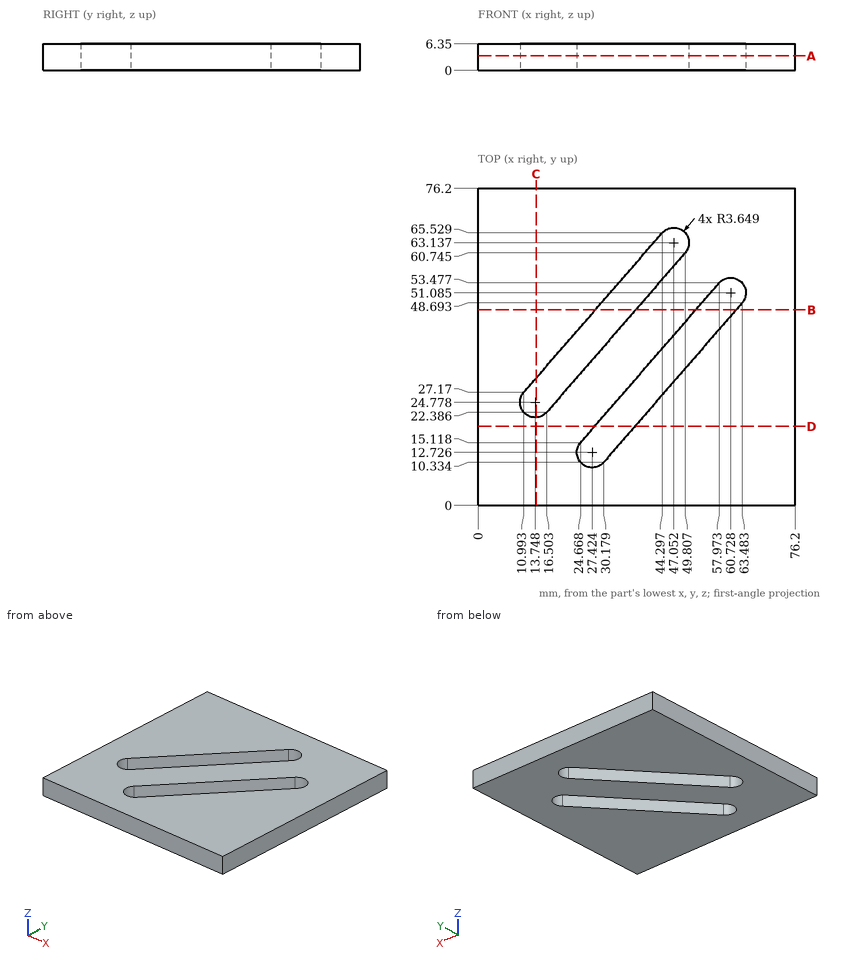
Study the drawing (mm; zero at the part's minimum x, y, z) and answer. Round coordinates to 2 decimals unless told otherwise and drop trailing zeros. Loops run counter-clockwise (first coordinate to the right, second up) from the corner with the lowest first, then second, coordinate; pieces in that order, holes last. Notation, with made-up numbers: (-25.5, 35) -> (20.5, 35) arc R17 cw to (20.5, 50) -> close; hole circle Ø1 at (45, 35.25). An arc over 180 degrees is marked (long way). Use one line per item in the form item = value.
1. The part is cut by section A-A on z = 3.5. Determine the outline of the cut face in (x, y) (1 decimal).
Answer key:
outline = (0, 0) -> (76.2, 0) -> (76.2, 76.2) -> (0, 76.2) -> close; hole (11, 27.2) arc R3.6 ccw to (16.5, 22.4) -> (49.8, 60.7) arc R3.6 ccw to (44.3, 65.5) -> close; hole (24.7, 15.1) arc R3.6 ccw to (30.2, 10.3) -> (63.5, 48.7) arc R3.6 ccw to (58, 53.5) -> close
2. Find the intervals of material crossed by probe 1 along X at (y, z) = (44.5, 5) (1 decimal); probe 2 along Y at (x, z) = (43.5, 3) (1 decimal); probe 3 along X at (y, z) = (33.5, 1.25) (1 decimal), in increasing order. Write a range as [from, to].
Answer key:
probe_1 = [0, 26], [35.7, 50.2], [59.8, 76.2]
probe_2 = [0, 25.7], [36.8, 53.5], [64.6, 76.2]
probe_3 = [0, 16.5], [26.2, 40.6], [50.3, 76.2]
3. The part is cut by section D-D on y = 19. Determine the outline of the cut face in (x, z).
Answer key:
outline = (0, 0) -> (28.04, 0) -> (28.04, 6.35) -> (0, 6.35) -> close; (37.7, 0) -> (76.2, 0) -> (76.2, 6.35) -> (37.7, 6.35) -> close
4. The part is cut by section C-C on x = 14. Determine the outline of the cut face in (y, z).
Answer key:
outline = (0, 0) -> (21.14, 0) -> (21.14, 6.35) -> (0, 6.35) -> close; (30.63, 0) -> (76.2, 0) -> (76.2, 6.35) -> (30.63, 6.35) -> close
5. The part is cut by section B-B on y = 47. Determine the outline of the cut face in (x, z).
Answer key:
outline = (0, 0) -> (28.21, 0) -> (28.21, 6.35) -> (0, 6.35) -> close; (37.87, 0) -> (52.35, 0) -> (52.35, 6.35) -> (37.87, 6.35) -> close; (62.01, 0) -> (76.2, 0) -> (76.2, 6.35) -> (62.01, 6.35) -> close
